Input: part model. Units: mm. Frame: model coordinates. A direction names the side the tool comes from. Round coordinates to 2 decimals unless told otherwise and drop trailing zeros. Loops run counter-clockwise (first coordinate to the right, second up) from the corner with the lowest first, then second, coordinate; pieces in that order, holes last. Notation, with made-up numbers: (-17.75, 76) - (15.25, 76) arc R27 ccw to (15.25, 109) - close; hole circle Ø3 at (38.5, 49). An arc over 180 degrees is marked (long way). Write each question's results on one line, items separated by ' | '.
from build123d import *

# Parameters (mm, degrees)
SKETCH2_R           = 20
BOSS_EXTRUDE1_DEPTH = 8
SKETCH3_R           = 1.5
CUT_EXTRUDE1_DEPTH  = 30.393876913
SKETCH4_R           = 12
CUT_EXTRUDE2_DEPTH  = 6.7


with BuildPart() as part:
    # Sketch2 → Boss-Extrude1 (new body)
    with BuildSketch(Plane(origin=(0, 0, 0), x_dir=(1, 0, 0), z_dir=(0, 1, 0))):
        with Locations(Location((0, 0, 0), (0, 0, 270))):
            Circle(SKETCH2_R)
    extrude(amount=BOSS_EXTRUDE1_DEPTH)

    # Sketch3 → Cut-Extrude1 (cut, through all)
    with BuildSketch(Plane(origin=(0, 8, 0), x_dir=(1, 0, 0), z_dir=(0, 1, 0))):
        with Locations(Location((0, 16, 0), (0, 0, 270))):
            Circle(SKETCH3_R)
        with Locations(Location((-16, 0, 0), (0, 0, 270))):
            Circle(SKETCH3_R)
        with Locations(Location((16, 0, 0), (0, 0, 270))):
            Circle(SKETCH3_R)
        with Locations(Location((0, -16, 0), (0, 0, 270))):
            Circle(SKETCH3_R)
    extrude(amount=-CUT_EXTRUDE1_DEPTH, mode=Mode.SUBTRACT)

    # Sketch4 → Cut-Extrude2 (cut)
    with BuildSketch(Plane(origin=(0, 8, -8), x_dir=(1, 0, 0), z_dir=(0, -1, 0))):
        with Locations(Location((0, 8, 0), (0, 0, 270))):
            Circle(SKETCH4_R)
    extrude(amount=CUT_EXTRUDE2_DEPTH, mode=Mode.SUBTRACT)


solid = part.part
1. Section query A-A, the plane z = 0. Output: boundary loops of the cut face in (x, y), plus the area to 3 significant figures.
Answer:
outline: (-20, 0) - (-17.5, 0) - (-17.5, 8) - (-20, 8) - close; (-14.5, 0) - (14.5, 0) - (14.5, 8) - (12, 8) - (12, 1.3) - (-12, 1.3) - (-12, 8) - (-14.5, 8) - close; (17.5, 0) - (20, 0) - (20, 8) - (17.5, 8) - close | area: 111 mm^2
2. Section query C-C, the plane x = -16. Output: boundary loops of the cut face in (y, z).
Answer:
outline: (0, -12) - (8, -12) - (8, -1.5) - (0, -1.5) - close; (0, 1.5) - (8, 1.5) - (8, 12) - (0, 12) - close
3. Contact query for flat-ended pins moving along their axis: pin 1 (12 mm diameter, centred on x = -0.5, z = 1, fed in from +Y); pin 2 (4 mm diameter, centred on y = 3, z = 7.5, fed in from -X); pin 3 (1.8 mm diameter, centred on x = -16, z = 0, fed in from -Y); pin 4 (4 mm diameter, centred on y = 3, z = -12, fed in from -X). Output: stop coordinate, or through.
Answer:
pin 1: y = 1.3 | pin 2: x = -19.23 | pin 3: through | pin 4: x = -17.32
4. Set-up query: faces 4 (the flat face through (0, 1.3, 0)), 5 (the flat face through (0, 0, 0)). Return all of +Z, -Z, +X, -X, +Y, -Y with unobstructed straight access to the full face (end or side cutting, diameter ignored); none if empty.
Answer:
face 4: +Y | face 5: +Z, -Z, +X, -X, -Y
5. Mould query, pull axis Z, two halves, no side actions, for faces 1 (the cylindrical face through (-15.55, 4.06, 1.43)), 2 (the flat face through (-9, 8, 9)), 3 (the cylindrical face through (-19.524, 3.944, -4.336)). Classes: pulls with the +Z half, pulls with the -Z half, needs draft (parallel to the pull), parting line crosses it, or undercut.
Answer:
face 1: undercut | face 2: needs draft | face 3: parting line crosses it
6. Section query B-B, the plane z = 16. Output: boundary loops of the cut face in (x, y).
Answer:
outline: (-12, 0) - (-1.5, 0) - (-1.5, 8) - (-12, 8) - close; (1.5, 0) - (12, 0) - (12, 8) - (1.5, 8) - close
7. Section query D-D, the plane y = 5. Output: boundary loops of the cut face in (x, z), plus the area to 3 significant figures.
Answer:
outline: circle Ø40 at (0, 0); hole circle Ø3 at (-16, 0); hole circle Ø24 at (0, 0); hole circle Ø3 at (0, -16); hole circle Ø3 at (0, 16); hole circle Ø3 at (16, 0) | area: 776 mm^2
8. Line query: line 1 (X direction, y = 3.25, z = 0); line 2 (X direction, y = 2.75, z = 16); line 3 (X direction, y = 2, z = -1). Output: solid intervals per line, ascending. Write a range as [from, to].
Answer:
line 1: [-20, -17.5], [-14.5, -12], [12, 14.5], [17.5, 20] | line 2: [-12, -1.5], [1.5, 12] | line 3: [-19.97, -17.12], [-14.88, -11.96], [11.96, 14.88], [17.12, 19.97]
